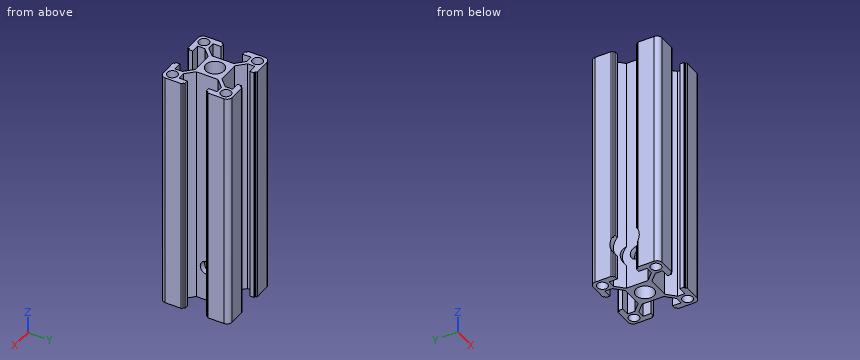
```python
from build123d import *

# Parameters (mm, degrees)
SKETCH_1_R               = 2.65
SKETCH_1_R_2             = 1.5
EXTRUDE_1_DEPTH          = 35
CUT_EXTRUDE_3_DEPTH      = 38.749172176
CUT_EXTRUDE_3_DEPTH_BACK = 38.749172176
SKETCH_5_R               = 2
SKETCH_6_R               = 4.25
CUT_EXTRUDE_4_DEPTH      = 39.946405572


with BuildPart() as part:
    # 草图1 → 凸台-拉伸1 (new, symmetric)
    with BuildSketch(Plane.XY):
        with BuildLine():
            Line((3.142893219, 3.85), (-3.142893219, 3.85))
            Line((-3.142893219, 3.85), (-5.5, 6.207106781))
            Line((-5.5, 6.207106781), (-5.5, 8.3))
            Line((-5.5, 8.3), (-3.1, 8.3))
            Line((-3.1, 8.3), (-3.1, 9.5))
            Line((-3.1, 9.5), (-3.6, 9.5))
            Line((-3.6, 9.5), (-3.6, 9.7))
            ThreePointArc((-3.6, 9.7), (-3.687867966, 9.912132034), (-3.9, 10))
            Line((-3.9, 10), (-8.5, 10))
            ThreePointArc((-8.5, 10), (-9.560660172, 9.560660172), (-10, 8.5))
            Line((-10, 8.5), (-10, 3.9))
            ThreePointArc((-10, 3.9), (-9.912132034, 3.687867966), (-9.7, 3.6))
            Line((-9.7, 3.6), (-9.5, 3.6))
            Line((-9.5, 3.6), (-9.5, 3.1))
            Line((-9.5, 3.1), (-8.3, 3.1))
            Line((-8.3, 3.1), (-8.3, 5.5))
            Line((-8.3, 5.5), (-6.207106781, 5.5))
            Line((-6.207106781, 5.5), (-3.85, 3.142893219))
            Line((-3.85, 3.142893219), (-3.85, -3.142893219))
            Line((-3.85, -3.142893219), (-6.207106781, -5.5))
            Line((-6.207106781, -5.5), (-8.3, -5.5))
            Line((-8.3, -5.5), (-8.3, -3.1))
            Line((-8.3, -3.1), (-9.5, -3.1))
            Line((-9.5, -3.1), (-9.5, -3.6))
            Line((-9.5, -3.6), (-9.7, -3.6))
            ThreePointArc((-9.7, -3.6), (-9.912132034, -3.687867966), (-10, -3.9))
            Line((-10, -3.9), (-10, -8.5))
            ThreePointArc((-10, -8.5), (-9.560660172, -9.560660172), (-8.5, -10))
            Line((-8.5, -10), (-3.9, -10))
            ThreePointArc((-3.9, -10), (-3.687867966, -9.912132034), (-3.6, -9.7))
            Line((-3.6, -9.7), (-3.6, -9.5))
            Line((-3.6, -9.5), (-3.1, -9.5))
            Line((-3.1, -9.5), (-3.1, -8.3))
            Line((-3.1, -8.3), (-5.5, -8.3))
            Line((-5.5, -8.3), (-5.5, -6.207106781))
            Line((-5.5, -6.207106781), (-3.142893219, -3.85))
            Line((-3.142893219, -3.85), (3.142893219, -3.85))
            Line((3.142893219, -3.85), (5.5, -6.207106781))
            Line((5.5, -6.207106781), (5.5, -8.3))
            Line((5.5, -8.3), (3.1, -8.3))
            Line((3.1, -8.3), (3.1, -9.5))
            Line((3.1, -9.5), (3.6, -9.5))
            Line((3.6, -9.5), (3.6, -9.7))
            ThreePointArc((3.6, -9.7), (3.687867966, -9.912132034), (3.9, -10))
            Line((3.9, -10), (8.5, -10))
            ThreePointArc((8.5, -10), (9.560660172, -9.560660172), (10, -8.5))
            Line((10, -8.5), (10, -3.9))
            ThreePointArc((10, -3.9), (9.912132034, -3.687867966), (9.7, -3.6))
            Line((9.7, -3.6), (9.5, -3.6))
            Line((9.5, -3.6), (9.5, -3.1))
            Line((9.5, -3.1), (8.3, -3.1))
            Line((8.3, -3.1), (8.3, -5.5))
            Line((8.3, -5.5), (6.207106781, -5.5))
            Line((6.207106781, -5.5), (3.85, -3.142893219))
            Line((3.85, -3.142893219), (3.85, 3.142893219))
            Line((3.85, 3.142893219), (6.207106781, 5.5))
            Line((6.207106781, 5.5), (8.3, 5.5))
            Line((8.3, 5.5), (8.3, 3.1))
            Line((8.3, 3.1), (9.5, 3.1))
            Line((9.5, 3.1), (9.5, 3.6))
            Line((9.5, 3.6), (9.7, 3.6))
            ThreePointArc((9.7, 3.6), (9.912132034, 3.687867966), (10, 3.9))
            Line((10, 3.9), (10, 8.5))
            ThreePointArc((10, 8.5), (9.560660172, 9.560660172), (8.5, 10))
            Line((8.5, 10), (3.9, 10))
            ThreePointArc((3.9, 10), (3.687867966, 9.912132034), (3.6, 9.7))
            Line((3.6, 9.7), (3.6, 9.5))
            Line((3.6, 9.5), (3.1, 9.5))
            Line((3.1, 9.5), (3.1, 8.3))
            Line((3.1, 8.3), (5.5, 8.3))
            Line((5.5, 8.3), (5.5, 6.207106781))
            Line((5.5, 6.207106781), (3.142893219, 3.85))
        make_face()
        Circle(SKETCH_1_R, mode=Mode.SUBTRACT)
        with Locations((-7.75, 7.75)):
            Circle(SKETCH_1_R_2, mode=Mode.SUBTRACT)
        with Locations((7.75, 7.75)):
            Circle(SKETCH_1_R_2, mode=Mode.SUBTRACT)
        with Locations((7.75, -7.75)):
            Circle(SKETCH_1_R_2, mode=Mode.SUBTRACT)
        with Locations((-7.75, -7.75)):
            Circle(SKETCH_1_R_2, mode=Mode.SUBTRACT)
    extrude(amount=EXTRUDE_1_DEPTH, both=True)

    # 草图5 → 切除-拉伸3 (cut, two sides: drawn at the far end of the back side and taken through both)
    with BuildSketch(Plane(origin=(0, 0, 0), x_dir=(0, 0, -1), z_dir=(1, 0, 0)).offset(-CUT_EXTRUDE_3_DEPTH_BACK)):
        with Locations(Location((25, 0, 0), (0, 0, 180))):
            Circle(SKETCH_5_R)
    extrude(amount=CUT_EXTRUDE_3_DEPTH + CUT_EXTRUDE_3_DEPTH_BACK, mode=Mode.SUBTRACT)

    # 草图6 → 切除-拉伸4 (cut, through all)
    with BuildSketch(Plane.ZY.offset(3.85)):
        with Locations((-25, 0)):
            Circle(SKETCH_6_R)
    extrude(amount=CUT_EXTRUDE_4_DEPTH, mode=Mode.SUBTRACT)


solid = part.part
```
Design review of the part built by this model. Coordinates are the model's own, in mm. Coordinates: 2 decimals unless noted, no trailing zeros. Order: outer loops, then holes, each group sorted by start corner. A loop starts at its lowest first (then second) coordinate and runs counter-clockwise, first axis right, second up. Notation, with made-up numbers: (44.25, -29.75) - (64.25, -29.75) arc R12 cw to (64.25, -18.75) - close; hole circle Ø5 at (50.5, 87). An arc over 180 degrees is marked (long way). One line per question, with ' | ' between items.
Q1. Consider section A-A, the plane x = 0. Give the boundary of the cut face in (y, z).
Answer key:
outline: (-3.85, -35) - (-2.65, -35) - (-2.65, 35) - (-3.85, 35) - close; (2.65, -35) - (3.85, -35) - (3.85, 35) - (2.65, 35) - close
Q2. Consider section C-C, the plane x = 7.25. Give the boundary of the cut face in (y, z), then the cut area to 3 significant figures.
Answer key:
outline: (-10, -35) - (-9.16, -35) - (-9.16, 35) - (-10, 35) - close; (-6.34, -35) - (-5.5, -35) - (-5.5, 35) - (-6.34, 35) - close; (5.5, -35) - (6.34, -35) - (6.34, 35) - (5.5, 35) - close; (9.16, -35) - (10, -35) - (10, 35) - (9.16, 35) - close | area: 234 mm2
Q3. Consider section B-B, the plane z = -25. Give the number of separate pieces and of enclosed holes in the cut face, then the cut area to 3 significant figures.
Answer key:
separate pieces: 2 | enclosed holes: 4 | area: 113 mm2
Q4. To check wall thickness, follow line 1 along Y through (x, z) = (7.75, 15.5); line 2 along Y through (x, z) = (0.25, -2.5); line 3 along Y through (x, z) = (-3.2, -25). State the ranges of each line that lie inside material, in increasing order.
Answer key:
line 1: y = -10 to -9.25, -6.25 to -5.5, 5.5 to 6.25, 9.25 to 10 | line 2: y = -3.85 to -2.64, 2.64 to 3.85 | line 3: y = -9.5 to -8.3, -3.91 to -2, 2 to 3.91, 8.3 to 9.5
Q5. Clearance check with flat-ended pins moving along their axes: pin 1 Ø0.6 at (y, z) = (9, 11.5) entering from -X; pin 2 Ø2.5 at (x, y) = (-7.75, -7.75) entering from -Z; pin 3 Ø0.6 at (x, z) = (3.5, -1.5) entering from -Y; pin 4 Ø1 at (y, z) = (0, -7) entering from -X. State where each tip first meets the part, or that it passes through.
Answer key:
pin 1: stops at x = -9.99 | pin 2: passes through | pin 3: stops at y = -9.98 | pin 4: stops at x = -3.85
